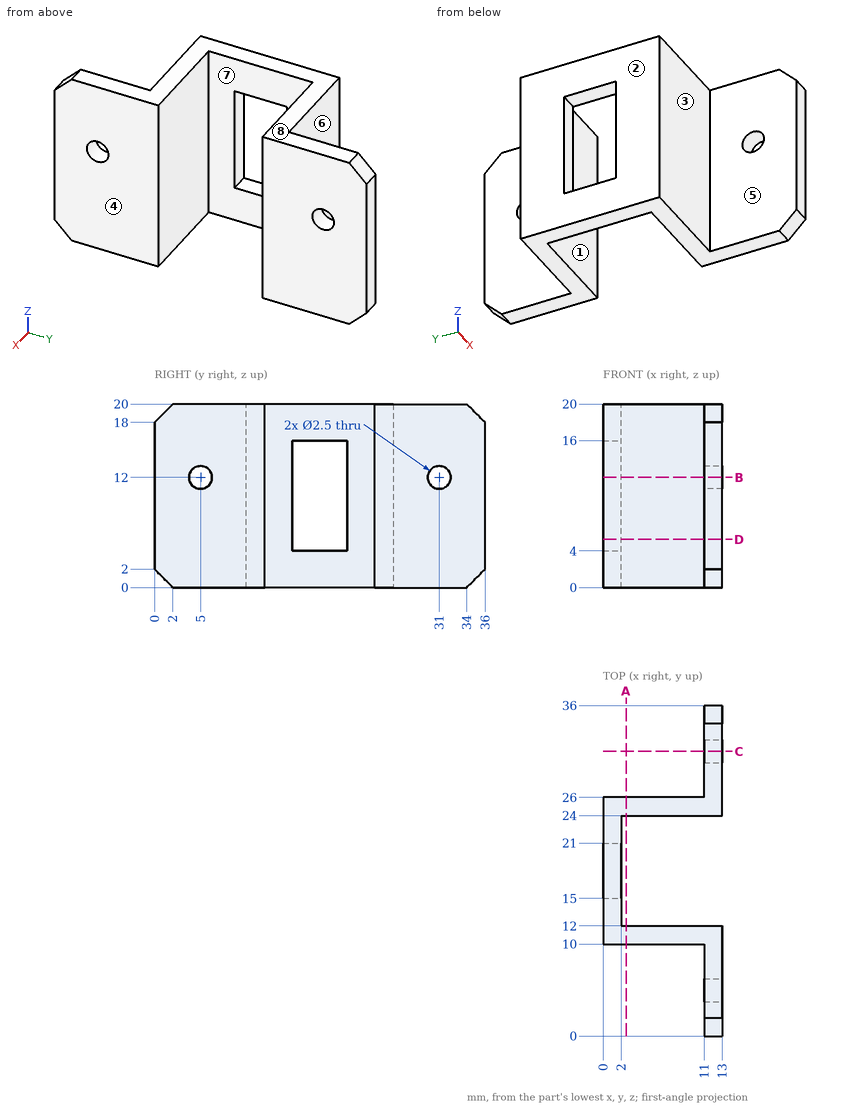
Could you check a few things on this drawing? It's one solid part, dimensions in mm from its lowest x, y, z. A direction names the side the tool comes from. Coordinates: 2 decimals unless noted, no trailing zeros. Order: outer loops, then holes, each group sorted by start corner. A loop starts at its lowest first (then second) coordinate and runs counter-clockwise, first axis right, second up. Notation, with made-up numbers: M 72,10.25 L 109,10.25 A30 cw 109,35.25 Z; hole C 22,14 d5. An arc over 180 degrees is marked long. Use one line per item in the form item = value. Start each with the question number.
1. Suppose I cut it at A-A on x = 2.5. Write out the boundary of the cut face in (y, z), then the cut area to 3 significant figures.
2. Please list where these lines run through material, in increasing order: line 1 (Y direction, x = 12, z = 12); line 2 (Z direction, x = 11.8, y = 5); line 3 (Y direction, x = 9, z = 11.5).
3. For pin 1 (1 mm diameter, centred on x = 1, z = 10.5, fed in from +Y); pin 2 (5 mm diameter, centred on y = 5.5, z = 12, fed in from -X); pin 3 (1 mm diameter, centred on x = 1.5, z = 13, fed in from -Y), each with a flat end and sliding along its axis, tell me the tip position at first contact or that it passes through.
4. Suppose I cut it at C-C on y = 31. Write out the boundary of the cut face in (x, z), then the cut area to 3 significant figures.
5. Suppose I cut it at D-D on z = 5.25. Write out the boundary of the cut face in (x, y).
6. Suppose I cut it at B-B on z = 12. Write out the boundary of the cut face in (x, y).
7. On a 3-axis mill with a long thin cutter (end or side, diameter ignored), from which of +Z, -Z, +X, -X, +Y, -Y can I reach the whole of each face in a straight line? I mean the marked faces 4, 5, 6, 7 and 8. Say none if no direction works.
8. We'd pull the mould along Y, two halves only. Please class the marked faces 1, 2 and 3: +Y half, -Y half, draft (parallel to the pull), parting line (faces both ways), or undercut.
Geometry says:
q1.outline = M 10,0 L 12,0 L 12,20 L 10,20 Z; M 24,0 L 26,0 L 26,20 L 24,20 Z
q1.area = 80.0 mm^2
q2.line_1 = 0 to 3.75, 6.25 to 12, 24 to 29.75, 32.25 to 36
q2.line_2 = 0 to 10.75, 13.25 to 20
q2.line_3 = 10 to 12, 24 to 26
q3.pin_1 = 26
q3.pin_2 = 11
q3.pin_3 = 10
q4.outline = M 11,0 L 13,0 L 13,10.75 L 11,10.75 Z; M 11,13.25 L 13,13.25 L 13,20 L 11,20 Z
q4.area = 35.0 mm^2
q5.outline = M 0,10 L 11,10 L 11,0 L 13,0 L 13,12 L 2,12 L 2,15 L 0,15 Z; M 0,21 L 2,21 L 2,24 L 13,24 L 13,36 L 11,36 L 11,26 L 0,26 Z
q6.outline = M 0,10 L 11,10 L 11,6.25 L 13,6.25 L 13,12 L 2,12 L 2,15 L 0,15 Z; M 0,21 L 2,21 L 2,24 L 13,24 L 13,29.75 L 11,29.75 L 11,26 L 0,26 Z; M 11,0 L 13,0 L 13,3.75 L 11,3.75 Z; M 11,32.25 L 13,32.25 L 13,36 L 11,36 Z
q7.face_4 = +Z, -Z, +X, +Y, -Y
q7.face_5 = +Z, -Z, -X, -Y
q7.face_6 = +Z, -Z, -X, +Y
q7.face_7 = +Z, -Z, +X
q7.face_8 = +Z, +X, -X, +Y, -Y
q8.face_1 = undercut
q8.face_2 = draft
q8.face_3 = -Y half
